Input: part model. Units: mm. Frame: model coordinates. A direction names the side the tool comes from. Coordinates: 2 decimals unless noted, no trailing zeros. Loops run counter-clockwise (first coordinate to the right, second up) from the corner with the lowest first, then second, coordinate; pieces in that order, holes last.
Item 1: Section C-C on x = -37.5. Return loops of the section in (y, z), and give its area (3 significant figures).
Item 2: Section D-D on y = 106. Return loops of the section in (x, z).
Item 3: Section B-B on y = 11. Return loops of the section in (x, z), and give its area (3 significant figures).
Item 4: Contact query for flat-ended pins moving along their axis: P1, Ø12, axis at x = 42, y = 24.5, coming from the +Z side; P2, Ø3, axis at x = 53.5, z = 11.5, coming from the -Y side; P3, Ø1.5, axis at y = 51.5, z = -5, coming from the -X side; P4, Ø4.5, axis at x = -15.5, y = 113.5, coming from the +Z side. Output: stop coordinate, or through.
Item 5: Ray query, line 1 along Y through (x, z) = (0, 6.75); line 2 along Y through (x, z) = (3, -7.75); line 3 along X through (y, z) = (-1, -7.75). Return the intervals inside material, ascending.
Item 6: Section A-A on z = 6.25. Return loops of the section in (x, y).
Item 7: Reachability of faces 5 (the flat face through (-33.5, 106, -8)), 6 (the cylindrical face through (-0.496, 73.723, -2.712)), 7 (the cylindrical face through (31.378, -60.328, 1.818)), 8 (the flat face through (0, 51, -7)) from +Z, -Z, +X, -X, +Y, -Y: full face, straight path, thin tool, end or side. Return the list, or none.
Item 8: Pull-direction query (Z, two-part tool) for faces 1 (the flat face through (44, -25, -4)), 2 (the flat face through (33.5, 107, -8)), 3 (the flat face through (-44, -25, -7)), 4 (the flat face through (14.93, 86.76, -5.5)); classes: released by +Z, released by -Z, zero draft, split by the parting line, or undercut.
```python
from build123d import *

# Parameters (mm, degrees)
BOSS_EXTRUDE1_DEPTH      = 15
BOSS_EXTRUDE1_DEPTH_BACK = 11
SKETCH1_R                = 68
SKETCH1_R_2              = 49
SKETCH2_W                = 43
SKETCH2_H                = 43
SKETCH2_R                = 18.5
BOSS_EXTRUDE2_DEPTH      = 11
SKETCH3_R                = 1.7
CUT_EXTRUDE1_DEPTH       = 140.929446508
SKETCH4_R                = 100
CUT_EXTRUDE2_DEPTH       = 5.5
SKETCH5_R                = 1.7
CUT_EXTRUDE3_DEPTH       = 140.929446508
SKETCH6_R                = 2.95
CUT_EXTRUDE4_DEPTH       = 3
CIRPATTERN1_COUNT        = 3
CUT_EXTRUDE5_DEPTH       = 3
CIRPATTERN2_COUNT        = 3


with BuildPart() as part:
    # Sketch1 → Boss-Extrude1 (new, two sides: drawn at the far end of the back side and taken through both)
    with BuildSketch(Plane.XY.offset(-BOSS_EXTRUDE1_DEPTH_BACK)):
        Circle(SKETCH1_R)
        Circle(SKETCH1_R_2, mode=Mode.SUBTRACT)
    extrude(amount=BOSS_EXTRUDE1_DEPTH + BOSS_EXTRUDE1_DEPTH_BACK)

    # Sketch2 → Boss-Extrude2 (add)
    # profile 1 of 6: a face of its own
    with BuildSketch(Plane(origin=(0, 0, -11), x_dir=(-1, 0, 0), z_dir=(0, 0, -1))):
        with BuildLine():
            Line((-33.5, 66.5), (-33.5, 93.149074069))
            ThreePointArc((-33.5, 93.149074069), (-38.168927278, 67.100269686), (-51.594405594, 44.294664592))
            ThreePointArc((-51.594405594, 44.294664592), (-34.722076366, 58.466891596), (-14.203872711, 66.5))
            Line((-14.203872711, 66.5), (-33.5, 66.5))
        make_face()
    # profile 2 of 6: a face of its own
    with BuildSketch(Plane(origin=(0, 0, -11), x_dir=(-1, 0, 0), z_dir=(0, 0, -1))):
        with BuildLine():
            ThreePointArc((-14.203872711, 66.5), (-34.722076366, 58.466891596), (-51.594405594, 44.294664592))
            Line((-51.594405594, 44.294664592), (-20.951913723, 44.294664592))
            ThreePointArc((-20.951913723, 44.294664592), (0, 49), (20.951913723, 44.294664592))
            Line((20.951913723, 44.294664592), (51.594405594, 44.294664592))
            ThreePointArc((51.594405594, 44.294664592), (34.722076366, 58.466891596), (14.203872711, 66.5))
            Line((14.203872711, 66.5), (-14.203872711, 66.5))
        make_face()
    # profile 3 of 6: a face of its own
    with BuildSketch(Plane(origin=(0, 0, -11), x_dir=(-1, 0, 0), z_dir=(0, 0, -1))):
        with BuildLine():
            ThreePointArc((51.594405594, 44.294664592), (38.168927278, 67.100269686), (33.5, 93.149074069))
            Line((33.5, 93.149074069), (33.5, 66.5))
            Line((33.5, 66.5), (14.203872711, 66.5))
            ThreePointArc((14.203872711, 66.5), (34.722076366, 58.466891596), (51.594405594, 44.294664592))
        make_face()
    # profile 4 of 6: a face of its own
    with BuildSketch(Plane(origin=(0, 0, -11), x_dir=(-1, 0, 0), z_dir=(0, 0, -1))):
        with BuildLine():
            ThreePointArc((14.203872711, 66.5), (0, 68), (-14.203872711, 66.5))
            Line((-14.203872711, 66.5), (14.203872711, 66.5))
        make_face()
    # profile 5 of 6: a face of its own
    with BuildSketch(Plane(origin=(0, 0, -11), x_dir=(-1, 0, 0), z_dir=(0, 0, -1))):
        with BuildLine():
            Line((-21.5, 76.5), (-21.5, 119.5))
            Line((-21.5, 119.5), (-33.5, 119.5))
            Line((-33.5, 119.5), (-33.5, 93.149074069))
            Line((-33.5, 93.149074069), (-33.5, 66.5))
            Line((-33.5, 66.5), (-14.203872711, 66.5))
            ThreePointArc((-14.203872711, 66.5), (0, 68), (14.203872711, 66.5))
            Line((14.203872711, 66.5), (33.5, 66.5))
            Line((33.5, 66.5), (33.5, 93.149074069))
            Line((33.5, 93.149074069), (33.5, 119.5))
            Line((33.5, 119.5), (21.5, 119.5))
            Line((21.5, 119.5), (21.5, 76.5))
            Line((21.5, 76.5), (-21.5, 76.5))
        make_face()
    # profile 6 of 6: a face of its own
    with BuildSketch(Plane(origin=(0, 0, -11), x_dir=(-1, 0, 0), z_dir=(0, 0, -1))):
        with Locations((0, 98)):
            Rectangle(SKETCH2_W, SKETCH2_H)
        with Locations((0, 98)):
            Circle(SKETCH2_R, mode=Mode.SUBTRACT)
    extrude(amount=-BOSS_EXTRUDE2_DEPTH)

    # Sketch3 → Cut-Extrude1 (cut, through all)
    with BuildSketch(Plane(origin=(0, 0, -11), x_dir=(-1, 0, 0), z_dir=(0, 0, -1))):
        with Locations((-15.5, 113.5)):
            Circle(SKETCH3_R)
        with Locations((15.5, 113.5)):
            Circle(SKETCH3_R)
        with Locations((15.5, 82.5)):
            Circle(SKETCH3_R)
        with Locations((-15.5, 82.5)):
            Circle(SKETCH3_R)
    extrude(amount=-CUT_EXTRUDE1_DEPTH, mode=Mode.SUBTRACT)

    # Sketch4 → Cut-Extrude2 (cut)
    with BuildSketch(Plane.XY):
        with Locations((0, 173.721812761)):
            Circle(SKETCH4_R)
    extrude(amount=-CUT_EXTRUDE2_DEPTH, mode=Mode.SUBTRACT)

    # Sketch5 → Cut-Extrude3 (cut, through all)
    with BuildSketch(Plane(origin=(0, 0, -11), x_dir=(-1, 0, 0), z_dir=(0, 0, -1))):
        with Locations((0, 61.5)):
            Circle(SKETCH5_R)
        with Locations((53.260562333, -30.75)):
            Circle(SKETCH5_R)
        with Locations((-53.260562333, -30.75)):
            Circle(SKETCH5_R)
        with Locations((0, 53)):
            Circle(SKETCH5_R)
        with Locations((45.899346401, -26.5)):
            Circle(SKETCH5_R)
        with Locations((-45.899346401, -26.5)):
            Circle(SKETCH5_R)
    extrude(amount=-CUT_EXTRUDE3_DEPTH, mode=Mode.SUBTRACT)

    # Sketch6 → Cut-Extrude4 (cut)
    with BuildSketch(Plane(origin=(0, 0, -11), x_dir=(-1, 0, 0), z_dir=(0, 0, -1))):
        with Locations((0, 61.5)):
            Circle(SKETCH6_R)
    cut_extrude4 = extrude(amount=-CUT_EXTRUDE4_DEPTH, mode=Mode.SUBTRACT)

    # CirPattern1: Cut-Extrude4 ×3 about axis
    cirpattern1_axis = Axis((0, 0, 0), (0, 0, 1))
    for i in range(1, CIRPATTERN1_COUNT):
        add(cut_extrude4.rotate(cirpattern1_axis, i * 360 / CIRPATTERN1_COUNT), mode=Mode.SUBTRACT)

    # Sketch7 → Cut-Extrude5 (cut)
    with BuildSketch(Plane(origin=(0, 0, -7), x_dir=(-1, 0, 0), z_dir=(0, 0, -1))):
        Polygon((-3.35, 44), (3.35, 44), (3.35, 53), (1.675, 50.098814897), (-1.675, 50.098814897), (-3.35, 53), align=None)
        Polygon((1.675, 50.098814897), (-1.675, 50.098814897), (-3.35, 53), (-1.675, 55.901185103), (1.675, 55.901185103), (3.35, 53), align=None)
    cut_extrude5 = extrude(amount=-CUT_EXTRUDE5_DEPTH, mode=Mode.SUBTRACT)

    # CirPattern2: Cut-Extrude5 ×3 about axis
    cirpattern2_axis = Axis((0, 0, 0), (0, 0, 1))
    for i in range(1, CIRPATTERN2_COUNT):
        add(cut_extrude5.rotate(cirpattern2_axis, i * 360 / CIRPATTERN2_COUNT), mode=Mode.SUBTRACT)


solid = part.part
```
Results found:
1. outline: (-56.73, -11) - (-31.54, -11) - (-31.54, 15) - (-56.73, 15) - close; (31.54, -11) - (68.98, -11) - (68.98, 0) - (56.73, 0) - (56.73, 15) - (31.54, 15) - close
1. area: 1,440 mm2
2. outline: (-33.5, -11) - (-16.68, -11) - (-16.68, -5.5) - (-33.5, -5.5) - close; (16.68, -11) - (33.5, -11) - (33.5, -5.5) - (16.68, -5.5) - close
3. outline: (-67.1, -11) - (-47.75, -11) - (-47.75, 15) - (-67.1, 15) - close; (47.75, -11) - (67.1, -11) - (67.1, 15) - (47.75, 15) - close
3. area: 1,010 mm2
4. P1: stops at z = 15
4. P2: stops at y = -43.82
4. P3: stops at x = -46.63
4. P4: stops at z = -5.5
5. line 1: y = -68 to -49, 49 to 51.3, 54.7 to 59.8, 63.2 to 68
5. line 2: y = -67.93 to -48.91, 48.91 to 79.74, 116.26 to 119.5
5. line 3: x = -67.99 to -48.99, 48.99 to 67.99
6. outline: circle Ø136 at (0, 0); hole circle Ø3.4 at (-53.26, -30.75); hole circle Ø98 at (0, 0); hole circle Ø3.4 at (-45.9, -26.5); hole circle Ø3.4 at (0, 53); hole circle Ø3.4 at (0, 61.5); hole circle Ø3.4 at (45.9, -26.5); hole circle Ø3.4 at (53.26, -30.75)
7. face 5: +Z, -Z, -X, +Y
7. face 6: +Z, +Y
7. face 7: +Z
7. face 8: none
8. face 1: undercut
8. face 2: zero draft
8. face 3: undercut
8. face 4: released by +Z
